from build123d import *

# Parameters (mm, degrees)
F1_DEPTH = 68
F2_W     = 3.5
F2_H     = 7.5
F3_DEPTH = 2
F4_R     = 2
F5_DEPTH = 25
F6_W     = 3.5
F6_H     = 3.5
F7_DEPTH = 3


with BuildPart() as f1:
    # F0 (on Right) → F1 (new body)
    with BuildSketch(Plane.YZ):
        with BuildLine():
            Line((-29.5, -9.5), (29.5, -9.5))
            ThreePointArc((29.5, -9.5), (31.62132, -8.62132), (32.5, -6.5))
            Line((32.5, -6.5), (32.5, 6.5))
            ThreePointArc((32.5, 6.5), (31.62132, 8.62132), (29.5, 9.5))
            Line((29.5, 9.5), (-29.5, 9.5))
            ThreePointArc((-29.5, 9.5), (-31.62132, 8.62132), (-32.5, 6.5))
            Line((-32.5, 6.5), (-32.5, -6.5))
            ThreePointArc((-32.5, -6.5), (-31.62132, -8.62132), (-29.5, -9.5))
        make_face()
    extrude(amount=F1_DEPTH)

    # F2 (on face) → F3 (cut)
    with BuildSketch(Plane.XY.offset(9.5)):
        with Locations((5.95, 20.95)):
            Rectangle(F2_W, F2_H)
    extrude(amount=-F3_DEPTH, mode=Mode.SUBTRACT)

    # F4 (on face) → F5 (cut)
    with BuildSketch(Plane(origin=(0, 0, 0), x_dir=(0, -1, 0), z_dir=(-1, 0, 0))):
        with Locations((8.5, 4)):
            Circle(F4_R)
    extrude(amount=-F5_DEPTH, mode=Mode.SUBTRACT)

    # F6 (on face) → F7 (join)
    with BuildSketch(Plane.XY.offset(7.5)):
        with Locations((5.95, 18.95)):
            Rectangle(F6_W, F6_H)
    extrude(amount=F7_DEPTH)


solid = f1.part
Source: CAD feature listing. Evaluate the final solid. Frame: model axes, mm. A direction names the side the tool comes from. Round coordinates to 2 decimals unless told otherwise and drop trailing zeros. Loops run counter-clockwise (first coordinate to the right, second up) from the corner with the lowest first, then second, coordinate; pieces in that order, holes last. Notation, with made-up numbers: (40, -27.5) - (69, -27.5) arc R22 ccw to (69, 9.5) - close; hole circle Ø1 at (70.25, 35). An arc over 180 degrees is marked (long way). Write item = value, one per line. Start each with the question number.
Item 1: Section query A-A on y = -8.5. Output: boundary loops of the cut face in (x, z).
Item 2: Section query C-C on y = -18. Output: boundary loops of the cut face in (x, z), plus the area to 3 significant figures.
Item 3: Reachability of faces 4 (the face through (4.2, 23, 9)), 5 (the face through (25, -8, 4)), 6 (the face through (33.52, -31.6, 8.64)) from +Z, -Z, +X, -X, +Y, -Y: full face, straight path, thin tool, end or side. Return the list, or none.
Item 4: First-contact query: pin 1 Ø2 at (y, z) = (-9, 4) entering from -X; pin 2 Ø1.5 at (x, z) = (6.5, 9) entering from +Y; pin 3 Ø1 at (x, z) = (6.5, 8.5) entering from -Y. Flat tips, straight axial feed; report the tip coordinate or a pass-through.
Item 5: Mould query, pull axis Z, two halves, no side actions, for faces 1 (the face through (6, 24.7, 9)), 2 (the face through (12.3, -6.9, 2.8)), 3 (the face through (6, 23, 7.5)). Classes: released by +Z, released by -Z, zero draft, split by the parting line, or undercut.
Item 6: Section query B-B on z = 4. Output: boundary loops of the cut face in (x, y), plus the area to 3 significant figures.
Item 7: Material intervals for line 1 (Z direction, x = 18.5, y = -8.5); line 2 (Z direction, x = 14.5, y = 0); line 3 (Y direction, x = 45, z = 8.25), sorted ascending.
Results list:
q1.outline = (0, -9.5) - (68, -9.5) - (68, 9.5) - (0, 9.5) - (0, 6) - (25, 6) - (25, 2) - (0, 2) - close
q2.outline = (0, -9.5) - (68, -9.5) - (68, 9.5) - (0, 9.5) - close
q2.area = 1,290 mm²
q3.face_4 = +Z
q3.face_5 = -X
q3.face_6 = +Z, +X, -X, -Y
q4.pin_1 = 25
q4.pin_2 = 31.94
q4.pin_3 = -32.1
q5.face_1 = zero draft
q5.face_2 = undercut
q5.face_3 = released by +Z
q6.outline = (0, -32.5) - (68, -32.5) - (68, 32.5) - (0, 32.5) - (0, -6.5) - (25, -6.5) - (25, -10.5) - (0, -10.5) - close
q6.area = 4,320 mm²
q7.line_1 = -9.5 to 2, 6 to 9.5
q7.line_2 = -9.5 to 9.5
q7.line_3 = -31.94 to 31.94
